Could you check a few things on this model? Use its own coordinates, in mm. Face numbers are marked on the shaded views. A direction names the side the tool comes from. Give positions to 0.01 mm unless a question says otherwise; leave off trailing zeros. Loops run counter-clockwise (first coordinate to the right, second up) from the corner with the lowest first, then second, coordinate; pieces in that order, holes last. Notation, with made-up numbers: M 83.5,-40 L 132.5,-40 A17 ccw 132.5,-23 Z; hole C 26,-40 d10. An arc over 180 degrees is marked long. Use a Markdown table: item, result. Add a question column.
1) Suppose I cut it at B-B on x = -22.5. List the corners of the cut face in (y, z) for me.
2) Which directions (+Z, -Z, +X, -X, +Y, -Y) give clear straight access to the entire face, cutting with the end or side of a thin tool? Please do the marked faces 1 and 2.
3) We'd pull the mould along X, two halves only. Please class the marked faces 3, 4, 5 and 6: +X half, -X half, draft (parallel to the pull), parting line (faces both ways), or undercut.
4) If I drill on line 1 along X through (y, z) = (14.9, 0.8) (3 decimals); line 2 along Y through (x, z) = (-8, 3.25); line 3 along X through (y, z) = (6.5, 7.75) (3 decimals), over which ranges is the centre line in solid material (lowest first)? Write a range as [from, to].
5) Suppose I cut it at D-D on y = 5.5. List the corners of the cut face in (x, z) for me (3 decimals), and give its area (3 significant figures).
6) Suppose I cut it at C-C on z = 8.25. List the corners of the cut face in (x, y) for me (3 decimals), and give its area (3 significant figures).
7) Will these pins go through, and if not, where does the flat tip stop? pin 1 Ø1.8 at (x, y) = (17.5, 6) entering from +Z; pin 2 Ø5 at (x, z) = (-10, 1.5) entering from -Y; pin 3 Ø0.7 at (x, y) = (-18.5, 24.5) entering from +Z; pin 4 Ø6 at (x, y) = (-1.5, 7) entering from +Z.
8) Suppose I cut it at A-A on y = 14.9. List the corners of the cut face in (x, z) for me (3 decimals).
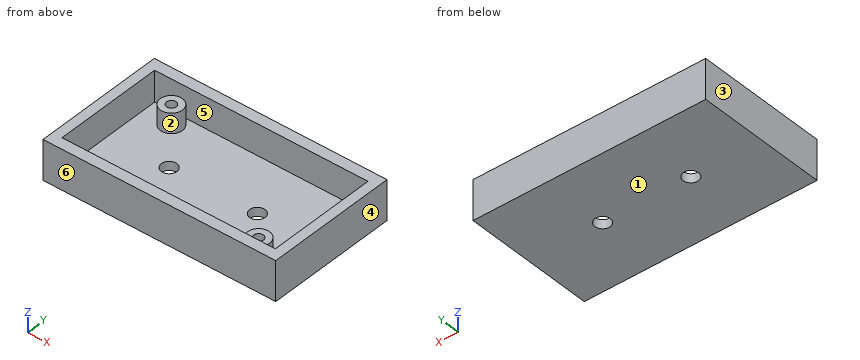
```python
from build123d import *

# Parameters (mm, degrees)
SKETCH_W        = 52.77
SKETCH_H        = 29.83
SKETCH_R        = 1.75
PAD_DEPTH       = 9
SKETCH001_W     = 48.37
SKETCH001_H     = 24.83
POCKET_DEPTH    = 7
SKETCH002_R     = 2.5
PAD001_DEPTH    = 4.5
SKETCH003_R     = 1.1
POCKET001_DEPTH = 3
SKETCH004_R     = 2.5
PAD002_DEPTH    = 4.5
SKETCH005_R     = 1.1
POCKET002_DEPTH = 3


with BuildPart() as part:
    # Sketch → Pad (new body)
    with BuildSketch(Plane.XY):
        with Locations((0, 14.915)):
            Rectangle(SKETCH_W, SKETCH_H)
        with Locations((-10.385, 14.9)):
            Circle(SKETCH_R, mode=Mode.SUBTRACT)
        with Locations((9.615, 14.9)):
            Circle(SKETCH_R, mode=Mode.SUBTRACT)
    extrude(amount=PAD_DEPTH)

    # Sketch001 (on Face8 of Pad) → Pocket (cut)
    with BuildSketch(Plane.XY.offset(9)):
        with Locations((0, 14.915)):
            Rectangle(SKETCH001_W, SKETCH001_H)
    extrude(amount=-POCKET_DEPTH, mode=Mode.SUBTRACT)

    # Sketch002 (on Face13 of Pocket) → Pad001 (join)
    with BuildSketch(Plane.XY.offset(2)):
        with Locations((-17.855, 24.33)):
            Circle(SKETCH002_R)
    extrude(amount=PAD001_DEPTH)

    # Sketch003 (on Face15 of Pad001) → Pocket001 (cut)
    with BuildSketch(Plane.XY.offset(6.5)):
        with Locations((-17.855, 24.33)):
            Circle(SKETCH003_R)
    extrude(amount=-POCKET001_DEPTH, mode=Mode.SUBTRACT)

    # Sketch004 (on Face13 of Pocket001) → Pad002 (join)
    with BuildSketch(Plane.XY.offset(2)):
        with Locations((17.855, 5.5)):
            Circle(SKETCH004_R)
    extrude(amount=PAD002_DEPTH)

    # Sketch005 (on Face16 of Pad002) → Pocket002 (cut)
    with BuildSketch(Plane.XY.offset(6.5)):
        with Locations((17.855, 5.5)):
            Circle(SKETCH005_R)
    extrude(amount=-POCKET002_DEPTH, mode=Mode.SUBTRACT)


solid = part.part
```
Answer block:
| question | item | result |
|---|---|---|
| 1 | outline | M 0,0 L 29.83,0 L 29.83,9 L 27.33,9 L 27.33,2 L 2.5,2 L 2.5,9 L 0,9 Z |
| 2 | face 1 | -Z, +X, -X, +Y, -Y |
| 2 | face 2 | +Z |
| 3 | face 3 | -X half |
| 3 | face 4 | +X half |
| 3 | face 5 | undercut |
| 3 | face 6 | draft |
| 4 | line 1 | x = [-26.385, -12.135], [-8.635, 7.865], [11.365, 26.385] |
| 4 | line 2 | y = [0, 2.5], [27.33, 29.83] |
| 4 | line 3 | x = [-26.385, -24.185], [24.185, 26.385] |
| 5 | outline | M -26.385,0 L 26.385,0 L 26.385,9 L 24.185,9 L 24.185,2 L 20.355,2 L 20.355,6.5 L 18.955,6.5 L 18.955,3.5 L 16.755,3.5 L 16.755,6.5 L 15.355,6.5 L 15.355,2 L -24.185,2 L -24.185,9 L -26.385,9 Z |
| 5 | area | 152 mm^2 |
| 6 | outline | M -26.385,0 L 26.385,0 L 26.385,29.83 L -26.385,29.83 Z; hole M -24.185,2.5 L 24.185,2.5 L 24.185,27.33 L -24.185,27.33 Z |
| 6 | area | 373 mm^2 |
| 7 | pin 1 | stops at z = 6.5 |
| 7 | pin 2 | stops at y = 0 |
| 7 | pin 3 | stops at z = 3.5 |
| 7 | pin 4 | stops at z = 2 |
| 8 | outline | M -26.385,0 L -12.135,0 L -12.135,2 L -24.185,2 L -24.185,9 L -26.385,9 Z; M -8.635,0 L 7.865,0 L 7.865,2 L -8.635,2 Z; M 11.365,0 L 26.385,0 L 26.385,9 L 24.185,9 L 24.185,2 L 11.365,2 Z |
